```python
from build123d import *

# Parameters (mm, degrees)
SKETCH_R        = 60
PAD_DEPTH       = 20
POCKET_DEPTH    = 16
SKETCH002_R     = 10
PAD001_DEPTH    = 52
SKETCH003_R     = 2.75
POCKET001_DEPTH = 52.001
SKETCH004_R     = 4.75
POCKET002_DEPTH = 5


with BuildPart() as part:
    # Sketch → Pad (new body)
    with BuildSketch(Plane.XY):
        with BuildLine():
            Line((0, 78), (-150, 78))
            Line((-150, 78), (-150, 48))
            ThreePointArc((-150, 48), (-143.193791, 28.97244), (-125.863464, 18.578583))
            ThreePointArc((-73.335895, -26.567772), (-93.676152, 2.897401), (-125.863464, 18.578583))
            ThreePointArc((-73.335895, -26.567772), (63.860341, -44.786794), (0, 78))
        make_face()
        Circle(SKETCH_R, mode=Mode.SUBTRACT)
    extrude(amount=PAD_DEPTH)

    # Sketch001 (on Face7 of Pad) → Pocket (cut)
    with BuildSketch(Plane(origin=(0, 0, 0), x_dir=(1, 0, 0), z_dir=(0, 0, -1))):
        with BuildLine():
            Line((-185.14, -73), (0, -73))
            ThreePointArc((0, -73), (72.609527, -7.540333), (15, 71.442284))
            Line((15, 71.442284), (-105.864687, 96.818997))
            Line((-105.864687, 96.818997), (-185.14, -73))
        make_face()
    extrude(amount=-POCKET_DEPTH, mode=Mode.SUBTRACT)

    # Sketch002 (on Face5 of Pocket) → Pad001 (join)
    with BuildSketch(Plane.XY.offset(20)):
        with Locations((-38.78477, 69.969577)):
            Circle(SKETCH002_R)
        with Locations((47.02282, 64.72136)):
            Circle(SKETCH002_R)
    extrude(amount=-PAD001_DEPTH)

    # Sketch003 (on Face22 of Pad001) → Pocket001 (cut, through all)
    with BuildSketch(Plane.XY.offset(20)):
        with Locations((-38.78477, 69.969577)):
            Circle(SKETCH003_R)
        with Locations((47.02282, 64.72136)):
            Circle(SKETCH003_R)
    extrude(amount=-POCKET001_DEPTH, mode=Mode.SUBTRACT)

    # Sketch004 (on Face20 of Pocket001) → Pocket002 (cut)
    with BuildSketch(Plane.XY.offset(20)):
        with Locations((-38.78477, 69.969577)):
            Circle(SKETCH004_R)
        with Locations((47.02282, 64.72136)):
            Circle(SKETCH004_R)
    extrude(amount=-POCKET002_DEPTH, mode=Mode.SUBTRACT)


solid = part.part
```
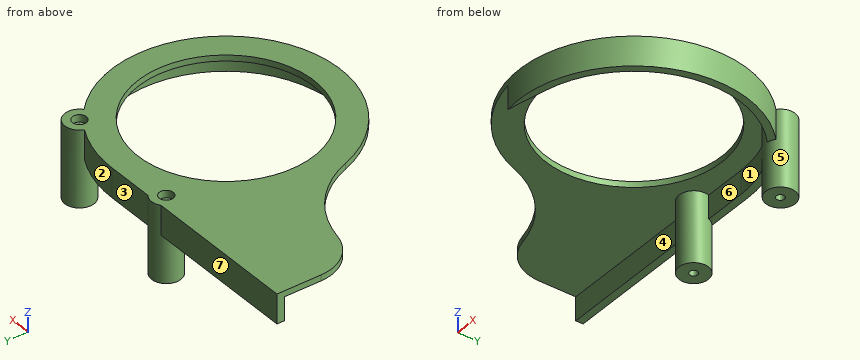
The model under review builds one solid part; all positions refer to its coordinate system, in mm. Face numbers are marked on the shaded views. A direction names the side the tool comes from. Coordinates: 2 decimals unless noted, no trailing zeros. Write each loop counter-clockwise with the first axis right and the second up, starting at its lowest first coordinate (ties: lowest second). Pieces come first, ordered by that corner, then holes. Notation, with made-up numbers: (26.5, 33) - (53.5, 33) arc R17 cw to (53.5, 43) - close; hole circle Ø6 at (-31.5, 7). An arc over 180 degrees is marked (long way). Write item = value, one per line.
(1) Consider section C-C, the plane z = -23.5. Give the boundary of the cut face in (x, y).
Result sheet:
outline = circle Ø20 at (-38.78, 69.97); circle Ø20 at (47.02, 64.72); hole circle Ø5.5 at (-38.78, 69.97); hole circle Ø5.5 at (47.02, 64.72)
(2) Consider section A-A, the plane y = -18. Give the boundary of the cut face in (x, z).
Result sheet:
outline = (-77.1, 16) - (-57.24, 16) - (-57.24, 20) - (-77.1, 20) - close; (57.24, 16) - (70.75, 16) - (70.75, 0) - (75.89, 0) - (75.89, 20) - (57.24, 20) - close
(3) For P1, Ø22, axis at x = -99, z = 8.5, coming from the +Y side; P2, Ø5, axis at y = 41, z = 9, coming from the -X side; P3, Ø1.5, axis at y = 18.5, z = 6.5, coming from the -X side; P4, Ø3, axis at x = 47, y = 64, coming from the -Z side, all flat-tipped, find the tip position at first contact; note any pin that passes through.
Result sheet:
P1 = 78
P2 = 58.62
P3 = 70.42
P4 = through
(4) For line 1 (X direction, y = 64.5, z = 10); line 2 (X direction, y = -0.5, z = 1); line 3 (Y direction, x = 49, z = 4.5), list the stretches that pass through material, from the lowest coordinate up. Write a range as [from, to].
Result sheet:
line_1 = [-47.16, -30.41], [34.19, 44.28], [49.76, 57.02]
line_2 = [73, 78]
line_3 = [-60.69, -54.11], [54.11, 62.81], [66.63, 74.52]
(5) Mouldability with a two-part tool opening along X and no side actions: class the marked faces 5, 6 and 7 as pulls with the +X half, pulls with the -X half, needs draft (parallel to the pull), parting line crosses it, or undercut.
Result sheet:
face_5 = undercut
face_6 = undercut
face_7 = needs draft
(6) Consider section B-B, the plane x = -2.5. Give the boundary of the cut face in (y, z).
Result sheet:
outline = (-77.96, 0) - (-75.12, 0) - (-75.12, 16) - (-59.95, 16) - (-59.95, 20) - (-77.96, 20) - close; (59.95, 16) - (73, 16) - (73, 0) - (78, 0) - (78, 20) - (59.95, 20) - close
(7) Machinability: for the marked faces 1, 2, 3 and 4, which of the approach directions +Z, -Z, +X, -X, +Y, -Y give a long, thin tool a straight path to every point of the face, cutting with its end or side? Answer none if there is none.
Result sheet:
face_1 = -Z
face_2 = +Z, -Z, +Y
face_3 = +Z, -Z, +X, +Y
face_4 = -Z, -X, -Y
(8) Consider section D-D, the plane y = 0. Give the boundary of the cut face in (x, z).
Result sheet:
outline = (-90.51, 16) - (-60, 16) - (-60, 20) - (-90.51, 20) - close; (60, 16) - (73, 16) - (73, 0) - (78, 0) - (78, 20) - (60, 20) - close
